For this review, use the dimensioned drawing (mm, ordinates from the lowest corner) and the shaded views. Give positions to 0.01 mm unless a question says otherwise; leave off trailing zeros. Loops run counter-clockwise (first coordinate to the right, second up) from the corner with the lowest first, then second, coordinate; pieces in that order, holes last. Notation, with made-up numbers: M 89.25,-31 L 145.25,-31 A14 ccw 145.25,-13 Z; hole C 25,25 d10. An arc over 180 degrees is marked long. Use a Markdown table: item, result. Add a question column.
(1) Draft analysis for pull direction X (two halves, no side actions). For the marked faces 1, 2 and 3, state which applies: pulls with the +X half, pulls with the -X half, needs draft (parallel to the pull), parting line crosses it, or undercut.
(2) Add section A-A, the plane x = 50.8. Give the boundary of the cut face in (y, z).
(3) Add section B-B, the plane y = 25.4. Give the boundary of the cut face in (x, z), then the cut area to 3 significant figures.
(4) For probe 1 along Y at (x, z) = (50.8, 2.5); probe 2 along Y at (x, z) = (4.5, 3.25); probe 3 along X at (y, z) = (20, 4.75), list the stretches that pass through material, from the lowest coordinate up.
(5) Add section C-C, the plane z = 1. Give the boundary of the cut face in (x, y), then the cut area to 3 significant figures.
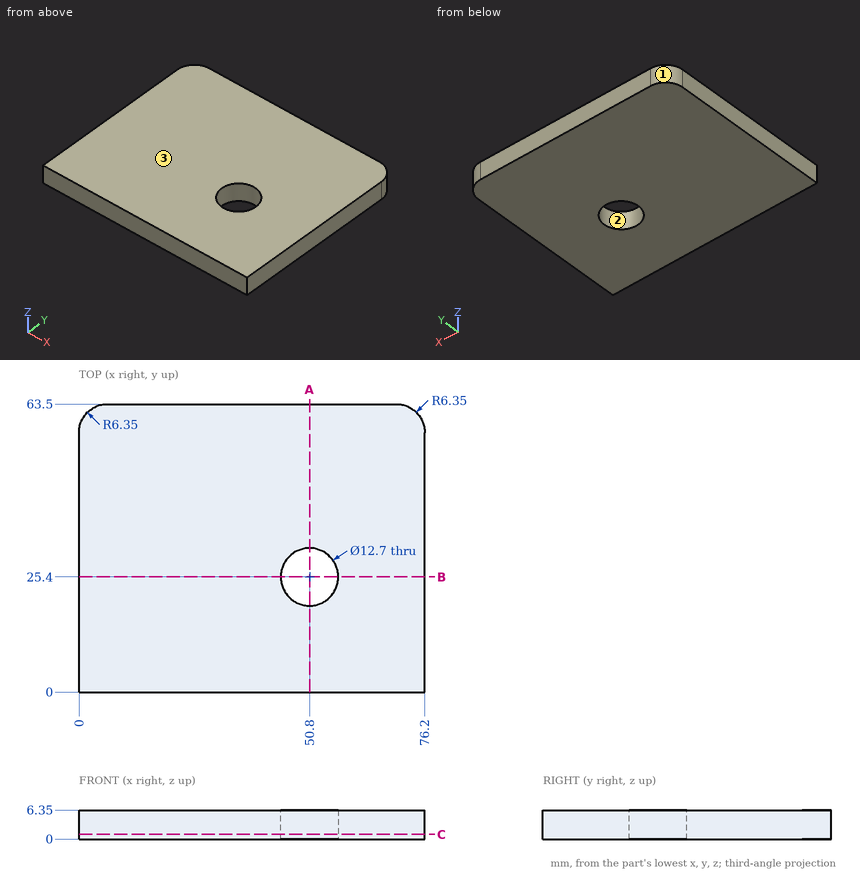
Established:
| question | item | result |
|---|---|---|
| 1 | face 1 | pulls with the -X half |
| 1 | face 2 | undercut |
| 1 | face 3 | needs draft |
| 2 | outline | M 0,0 L 19.05,0 L 19.05,6.35 L 0,6.35 Z; M 31.75,0 L 63.5,0 L 63.5,6.35 L 31.75,6.35 Z |
| 3 | outline | M 0,0 L 44.45,0 L 44.45,6.35 L 0,6.35 Z; M 57.15,0 L 76.2,0 L 76.2,6.35 L 57.15,6.35 Z |
| 3 | area | 403 mm^2 |
| 4 | probe 1 | 0 to 19.05, 31.75 to 63.5 |
| 4 | probe 2 | 0 to 63.22 |
| 4 | probe 3 | 0 to 47.46, 54.14 to 76.2 |
| 5 | outline | M 0,0 L 76.2,0 L 76.2,57.15 A6.35 ccw 69.85,63.5 L 6.35,63.5 A6.35 ccw 0,57.15 Z; hole C 50.8,25.4 d12.7 |
| 5 | area | 4,690 mm^2 |
